For this review, take the finished solid that the model builds, in its own axes (mm). A direction names the side the tool comes from. Coordinates: 2 decimals unless noted, no trailing zeros. Loops run counter-clockwise (first coordinate to the right, second up) from the corner with the lowest first, then second, coordinate; pieces in that order, holes last. Notation, with made-up numbers: M 35,83 L 52,83 A9 cw 52,97 Z; hole C 63.25,7 d8. An arc over 180 degrees is marked long. Answer as a JSON object with one key per item and string values. Group by question number.
Item 1: Wall thickness on L1, parallel to X at y = 9.5, z = 155.5; L2, parallel to Y at x = 32, z = 69; L3, parallel to Z at x = 20, y = 64: over which ranges is each line inside the solid? List them lowest first. Write a range as from..to.
Item 2: Add section A-A (y = 22). State the section outline as (x, z) points.
Item 3: Add section B-B (z = 99). State the section outline as (x, y) points, then the cut area to 3 significant figures.
Item 4: Insertion check: pin 1 (1.7 mm diameter, centred on x = 1, z = 14.5, fed in from +Y); pin 2 (25 mm diameter, centred on x = 47, y = 53, fed in from +Z); pin 3 (1.7 mm diameter, centred on x = 157, z = 182, fed in from +Y). Each pin has a flat end and moves straight along its axis. Give the tip position at first contact, or say it passes through.
Item 5: Add section D-D (y = 73.5). State the section outline as (x, z) points.
Item 6: Tool access review of faces 5 (the face through (0, 13, 111)), 6 (the face through (156.7, 35, 13.1)), 7 (the face through (155.892, 10, 113)): name each direction out of +Z, -Z, +X, -X, +Y, -Y from which nothing blocks a thin tool from reaching the whole face with its end or side.
Item 7: Mouldability with a two-part tool opening along Z and no side actions: class faces 1 (the face through (78, 40, 0)), 2 (the face through (78, -1.588, 122)), 3 (the face through (0.8, 35, 13.1)), 4 (the face through (0.78, 40.58, 16.37)) as +Z half, -Z half, draft (parallel to the pull), parting line (faces both ways), or undercut.
Item 8: Add section C-C (x = 17.5). State the section outline as (y, z) points, then the cut area to 3 significant figures.
from build123d import *

# Parameters (mm, degrees)
F0_W      = 157.48
F0_H      = 82.55
F1_DEPTH  = 1.5875
F2_W      = 157.48
F2_H      = 241.3
F3_DEPTH  = 1.5875
F4_W      = 19.304
F4_H      = 241.3
F5_DEPTH  = 1.5875
F7_W      = 24.9697454274
F7_H      = 239.1684796894
F8_DEPTH  = 1.5875
F10_W     = 19.304
F10_H     = 241.3
F11_DEPTH = 1.5875
F13_DEPTH = 1.5875
F15_DEPTH = 1.5875


with BuildPart() as f1:
    # F0 (on Top) → F1 (new body)
    with BuildSketch(Plane.XY):
        with Locations((78.74, 41.275)):
            Rectangle(F0_W, F0_H)
    extrude(amount=F1_DEPTH)

    # F2 (on Front) → F3 (join)
    with BuildSketch(Plane.XZ):
        with Locations((78.74, 120.65)):
            Rectangle(F2_W, F2_H)
    extrude(amount=F3_DEPTH)

    # F4 (on Right) → F5 (join)
    with BuildSketch(Plane.YZ):
        with Locations((9.652, 120.65)):
            Rectangle(F4_W, F4_H)
    extrude(amount=F5_DEPTH)

    # F10 (on 3pt) → F11 (join)
    with BuildSketch(Plane.YZ.offset(157.48)):
        with Locations((9.652, 120.65)):
            Rectangle(F10_W, F10_H)
    extrude(amount=-F11_DEPTH)

    # F12 (on 3pt) → F13 (join)
    with BuildSketch(Plane.YZ.offset(157.48)):
        Polygon((63.5, 0), (0, 45.3571428571), (0, 38.1), (53.34, 0), align=None)
    extrude(amount=-F13_DEPTH)

    # F14 (on Right) → F15 (join)
    with BuildSketch(Plane.YZ):
        Polygon((63.5, 0), (0, 45.3571428571), (0, 38.1), (53.34, 0), align=None)
    extrude(amount=F15_DEPTH)


with BuildPart() as f8:
    # F7 (on 3pt) → F8 (new body)
    with BuildSketch(Plane.YZ.offset(157.48)):
        with Locations((12.4848727137, 121.3677601772)):
            Rectangle(F7_W, F7_H)
    extrude(amount=-F8_DEPTH)


solid = f1.part
From the geometry:
{
 "1": {"L1": "x = 0..1.59, 155.89..157.48", "L2": "y = -1.59..0", "L3": "z = 0..1.59"},
 "2": {"outline": "M 0,0 L 157.48,0 L 157.48,1.59 L 0,1.59 Z; M 0,22.39 L 1.59,22.39 L 1.59,29.64 L 0,29.64 Z; M 155.89,22.39 L 157.48,22.39 L 157.48,29.64 L 155.89,29.64 Z"},
 "3": {"outline": "M 0,-1.59 L 157.48,-1.59 L 157.48,19.3 L 155.89,19.3 L 155.89,0 L 1.59,0 L 1.59,19.3 L 0,19.3 Z", "area": "311 mm²"},
 "4": {"pin 1": "stops at y = 44.39", "pin 2": "stops at z = 1.59", "pin 3": "stops at y = 19.3"},
 "5": {"outline": "M 0,0 L 157.48,0 L 157.48,1.59 L 0,1.59 Z"},
 "6": {"face 5": "+Z, -Z, -X, +Y, -Y", "face 6": "+X, -X", "face 7": "+Z, +Y"},
 "7": {"face 1": "-Z half", "face 2": "draft", "face 3": "undercut", "face 4": "+Z half"},
 "8": {"outline": "M -1.59,0 L 82.55,0 L 82.55,1.59 L 0,1.59 L 0,241.3 L -1.59,241.3 Z", "area": "514 mm²"}
}
